from build123d import *

# Parameters (mm, degrees)
BOSS_EXTRUDE1_DEPTH     = 3
SKETCH2_R               = 4
SKETCH2_W               = 200
SKETCH2_H               = 4
BOSS_EXTRUDE2_DEPTH     = 5.2
CUT_EXTRUDE3_DEPTH      = 149.751605033
CUT_EXTRUDE3_DEPTH_BACK = 149.751605033
SKETCH4_W               = 200.256598964
SKETCH4_H               = 45.821107358
CUT_EXTRUDE4_DEPTH      = 149.886668308
CUT_EXTRUDE4_DEPTH_BACK = 149.886668308
SKETCH5_W               = 32
SKETCH5_H               = 27.954907266
FILLET1_R               = 1
FILLET2_R               = 4
FILLET3_R               = 8
FILLET4_R               = 8


with BuildPart() as part:
    # Sketch1 → Boss-Extrude1 (new body)
    with BuildSketch(Plane.XY):
        with BuildLine():
            ThreePointArc((0, -110), (-59.410296816, -92.57654472), (-100, -45.82575695))
            Line((-100, -45.82575695), (-100, -110))
            Line((-100, -110), (0, -110))
        make_face()
        with BuildLine():
            ThreePointArc((0, -95), (-51.308892705, -79.95247044), (-86.363636364, -39.576790093))
            Line((-86.363636364, -39.576790093), (-100, -45.82575695))
            ThreePointArc((-100, -45.82575695), (-59.410296816, -92.57654472), (0, -110))
            Line((0, -110), (0, -95))
        make_face()
        with BuildLine():
            Line((100, -45.82575695), (86.363636364, -39.576790093))
            ThreePointArc((86.363636364, -39.576790093), (51.308892705, -79.95247044), (0, -95))
            Line((0, -95), (0, -110))
            ThreePointArc((0, -110), (59.410296816, -92.57654472), (100, -45.82575695))
        make_face()
        with BuildLine():
            Line((100, -110), (100, -45.82575695))
            ThreePointArc((100, -45.82575695), (59.410296816, -92.57654472), (0, -110))
            Line((0, -110), (100, -110))
        make_face()
    extrude(amount=BOSS_EXTRUDE1_DEPTH)

    # Sketch2 → Boss-Extrude2 (add)
    with BuildSketch(Plane.XY.offset(3)):
        with Locations((-54.25, -93.963756311)):
            Circle(SKETCH2_R)
        with Locations((54.25, -93.963756311)):
            Circle(SKETCH2_R)
        with Locations((0, -108)):
            Rectangle(SKETCH2_W, SKETCH2_H)
    extrude(amount=BOSS_EXTRUDE2_DEPTH)

    # Sketch4 → Cut-Extrude3 (cut, two sides: drawn at the far end of the back side and taken through both)
    with BuildSketch(Plane.XY.offset(3).offset(-CUT_EXTRUDE3_DEPTH_BACK)):
        with Locations((0.128299482, -59.134539055)):
            Rectangle(SKETCH4_W, SKETCH4_H)
    extrude(amount=CUT_EXTRUDE3_DEPTH + CUT_EXTRUDE3_DEPTH_BACK, mode=Mode.SUBTRACT)

    # Sketch5 → Cut-Extrude4 (cut, two sides: drawn at the far end of the back side and taken through both)
    with BuildSketch(Plane(origin=(0, 0, 0), x_dir=(-1, 0, 0), z_dir=(0, 0, -1)).offset(-CUT_EXTRUDE4_DEPTH_BACK)):
        with Locations((-84, -96.022546367)):
            Rectangle(SKETCH5_W, SKETCH5_H)
        with Locations((84, -96.022546367)):
            Rectangle(SKETCH5_W, SKETCH5_H)
    extrude(amount=CUT_EXTRUDE4_DEPTH + CUT_EXTRUDE4_DEPTH_BACK, mode=Mode.SUBTRACT)

    # Fillet1
    fillet1_edges = [part.edges().sort_by_distance(p)[0] for p in [
        (50.25, -93.963756311, 3),
        (-58.25, -93.963756311, 3),
    ]]
    fillet(fillet1_edges, radius=FILLET1_R)

    # Fillet2
    fillet2_edges = [part.edges().sort_by_distance(p)[0] for p in [
        (0, -106, 3),
    ]]
    fillet(fillet2_edges, radius=FILLET2_R)

    # Mirror1: part across plane


with BuildPart() as part_1:
    add(part.part)
    add(part.part.mirror(Plane.XY.offset(8.2)))

    # Fillet3
    # the kernel refuses this fillet: 8 mm, written as the material it takes off along each edge
    with BuildSketch(Plane(origin=(-68, -110, -20), x_dir=(1, 0, 0), z_dir=(0, 0, 1)), Plane(origin=(68, -110, 36.4), x_dir=(-1, 0, 0), z_dir=(0, 0, -1))) as fillet3_piece_1:
        with BuildLine():
            CenterArc((FILLET3_R, FILLET3_R), FILLET3_R, 180, 90)
            Line((0, FILLET3_R), (0, 0))
            Line((0, 0), (FILLET3_R, 0))
        make_face()
    extrude(amount=56.4, mode=Mode.SUBTRACT)
    with BuildSketch(Plane(origin=(-68, -82.045092734, -6.6), x_dir=(1, 0, 0), z_dir=(0, 0, 1)), Plane(origin=(68, -82.045092734, 36.4), x_dir=(-1, 0, 0), z_dir=(0, 0, -1))) as fillet3_piece_2:
        with BuildLine():
            CenterArc((FILLET3_R, -FILLET3_R), FILLET3_R, 90, 90)
            Line((0, -FILLET3_R), (0, 0))
            Line((0, 0), (FILLET3_R, 0))
        make_face()
    extrude(amount=43, mode=Mode.SUBTRACT)
    with BuildSketch(Plane(origin=(68, -82.045092734, -20), x_dir=(-1, 0, 0), z_dir=(0, 0, 1)), Plane(origin=(-68, -82.045092734, 23), x_dir=(1, 0, 0), z_dir=(0, 0, -1))) as fillet3_piece_3:
        with BuildLine():
            CenterArc((FILLET3_R, FILLET3_R), FILLET3_R, 180, 90)
            Line((0, FILLET3_R), (0, 0))
            Line((0, 0), (FILLET3_R, 0))
        make_face()
    extrude(amount=43, mode=Mode.SUBTRACT)

    # Fillet4
    fillet4_edges = [part_1.edges().sort_by_distance(p)[0] for p in [
        (-47.891572936, -82.045092734, 14.9),
        (47.891572936, -82.045092734, 14.9),
        (-47.891572936, -82.045092734, 1.5),
        (47.891572936, -82.045092734, 1.5),
    ]]
    fillet(fillet4_edges, radius=FILLET4_R)


solid = part_1.part
Geometry check sheet. Reference: the model listing, model coordinates, mm. A direction names the side the tool comes from. Round coordinates to 2 decimals unless told otherwise and drop trailing zeros. Loops run counter-clockwise (first coordinate to the right, second up) from the corner with the lowest first, then second, coordinate; pieces in that order, holes last. Notation, with made-up numbers: (33, 55.25) - (40, 55.25) arc R24 cw to (40, 71.25) - close; hole circle Ø6 at (65, 79.25). An arc over 180 degrees is marked (long way). One line per question, with ' | ' between items. Start each with the question number.
1. Draft check along X on faces 1 (the face through (-68, -96, 1)), 2 (the face through (0.952, -104.797, 4.141)), 3 (the face through (48, -82.3, 14.9)). Enter one of: released by +X, released by -X, zero draft, split by the parting line, or undercut.
2. Cross-section at D-D on x = 35. Record the cut outline in (y, z).
3. Depth check by flat-ended pin: pin 1 (3 mm diameter, centred on y = -88, z = 6.5, fed in from +X); pin 2 (2 mm diameter, centred on y = -106, z = 11.5, fed in from -X); pin 3 (2.5 mm diameter, centred on x = -20, z = 8.5, fed in from +Y); pin 4 (5 mm diameter, centred on x = 25.5, z = 11, fed in from +Y). Enter the tip coordinate at first touch or a pass-through.
4. Tool access check on faces 4 (the face through (-68, -96, 15)), 5 (the face through (48, -82.3, 1.5)). Record the directions out of +Z, -Z, +X, -X, +Y, -Y that give a thin tool (end or side, any length) a straight path to the whole face; none if there is none.
5. Scan lines: line 1 (Z direction, x = 42.5, y = -98.75); line 2 (X direction, y = -95.75, z = 9.5); line 3 (Y direction, x = -56.5, z = 4.5). Record each from-to range of solid material in increasing order. Write a range as [from, to].
6. Cross-section at B-B on z = 11. Record the cut outline in (x, y).
7. Cross-section at C-C on x = -36. Record the cut outline in (y, z).
8. Cross-section at A-A on x = -54.25. Record the cut outline in (y, z).
Taken from the geometry:
1) face 1: released by -X | face 2: zero draft | face 3: undercut
2) outline: (-110, 0) - (-88.32, 0) - (-88.32, 3) - (-102, 3) arc R4 cw to (-106, 7) - (-106, 9.4) arc R4 cw to (-102, 13.4) - (-88.32, 13.4) - (-88.32, 16.4) - (-110, 16.4) - close
3) pin 1: through | pin 2: x = -67.38 | pin 3: y = -105.98 | pin 4: y = -91.32
4) face 4: +Z, -Z, -X, +Y, -Y | face 5: +Z, -Z, +Y
5) line 1: [0, 3], [13.4, 16.4] | line 2: [-57.83, -50.67], [50.67, 57.83] | line 3: [-110, -105.12], [-97.27, -90.66]
6) outline: (-67.11, -105.67) arc R8 ccw to (-60, -110) - (60, -110) arc R8 ccw to (67.11, -105.67) - close; circle Ø8 at (-54.25, -93.96); circle Ø8 at (54.25, -93.96)
7) outline: (-110, 0) - (-87.91, 0) - (-87.91, 3) - (-102, 3) arc R4 cw to (-106, 7) - (-106, 9.4) arc R4 cw to (-102, 13.4) - (-87.91, 13.4) - (-87.91, 16.4) - (-110, 16.4) - close
8) outline: (-110, 0) - (-82.05, 0) - (-82.05, 3) - (-88.96, 3) arc R1 cw to (-89.96, 4) - (-89.96, 12.4) arc R1 cw to (-88.96, 13.4) - (-82.05, 13.4) - (-82.05, 16.4) - (-110, 16.4) - close; hole (-106, 7) arc R4 ccw to (-102, 3) - (-98.96, 3) arc R1 ccw to (-97.96, 4) - (-97.96, 12.4) arc R1 ccw to (-98.96, 13.4) - (-102, 13.4) arc R4 ccw to (-106, 9.4) - close
